Geometry: see drawing. Coordinates: mm, zero at the bounding-box minimum. Give positions to 0.01 mm unless a question says otherwise; leave off trailing zeros. Write each loop counter-clockwise with the first axis right and the second up, starting at its lowest first coordinate (ties: lowest second). Pieces come first, ordered by that corner, then holes. Notation, with made-up numbers: (-29.5, 66) -> (-1.5, 66) arc R22 cw to (-1.5, 79) -> close; hole circle Ø5 at (26, 41). An arc over 180 degrees is marked (long way). Answer as a JSON object with one key per item and string values. Group by question number.
Item 1: Section query A-A on x = 250. Return the cut outline in (y, z), plus the area to 3 significant figures.
Item 2: Section query C-C on z = 15. Return the cut outline in (x, y).
Item 3: Ray query, probe 1 along X at (y, z) = (2.75, 105); probe 2 along Z at (x, y) = (250, 1.4); probe 3 along Z at (x, y) = (15, 4.5). Return the intervals inside material, ascending. Write a range as from..to.
Item 4: Section query D-D on y = 2. Return the cut outline in (x, z), plus the area to 3 significant figures.
Item 5: Section query B-B on x = 15. Return the cut outline in (y, z), plus the area to 3 significant figures.
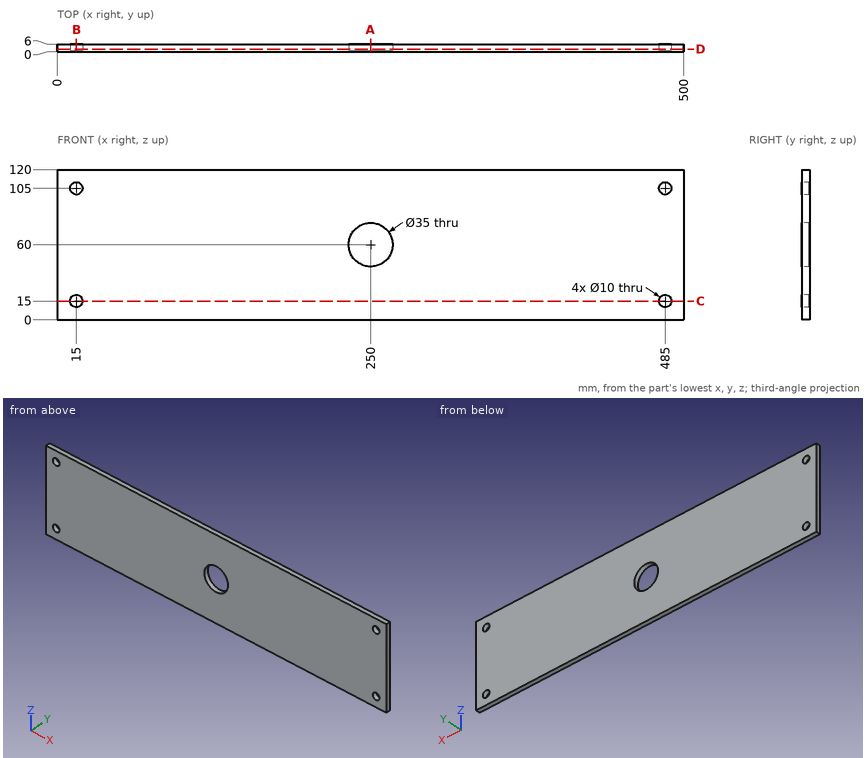
Worked answers:
{
 "1": {"outline": "(0, 0) -> (6, 0) -> (6, 42.5) -> (0, 42.5) -> close; (0, 77.5) -> (6, 77.5) -> (6, 120) -> (0, 120) -> close", "area": "510 mm^2"},
 "2": {"outline": "(0, 0) -> (10, 0) -> (10, 6) -> (0, 6) -> close; (20, 0) -> (480, 0) -> (480, 6) -> (20, 6) -> close; (490, 0) -> (500, 0) -> (500, 6) -> (490, 6) -> close"},
 "3": {"probe 1": "0..10, 20..480, 490..500", "probe 2": "0..42.5, 77.5..120", "probe 3": "0..10, 20..100, 110..120"},
 "4": {"outline": "(0, 0) -> (500, 0) -> (500, 120) -> (0, 120) -> close; hole circle Ø10 at (15, 15); hole circle Ø10 at (15, 105); hole circle Ø35 at (250, 60); hole circle Ø10 at (485, 15); hole circle Ø10 at (485, 105)", "area": "58,700 mm^2"},
 "5": {"outline": "(0, 0) -> (6, 0) -> (6, 10) -> (0, 10) -> close; (0, 20) -> (6, 20) -> (6, 100) -> (0, 100) -> close; (0, 110) -> (6, 110) -> (6, 120) -> (0, 120) -> close", "area": "600 mm^2"}
}
